Verification items for the finished model (mm, model axes). Coordinates: 2 decimals unless noted, no trailing zeros. Write each loop counter-clockwise with the first axis right and the second up, starting at its lowest first coordinate (ties: lowest second). Pieces come first, ordered by that corner, then holes. Notation, with made-up numbers: (67.5, 79) - (106.5, 79) arc R7 cw to (106.5, 92) - close; hole circle Ø1 at (44, -20.5). An arc over 180 degrees is marked (long way). Use CSV: the item, a comma, the result in double quotes. Start each with the question number.
```python
from build123d import *

# Parameters (mm, degrees)
F0_R     = 15
F0_R_2   = 22.5
F1_DEPTH = 15
F2_DEPTH = 15.001
F3_R     = 3
F4_DEPTH = 25


with BuildPart() as f1:
    # F0 (on Front) → F1 (new body)
    with BuildSketch(Plane.XZ):
        Circle(F0_R)
        Circle(F0_R_2)
        Circle(F0_R, mode=Mode.SUBTRACT)
    extrude(amount=-F1_DEPTH)

    # F0 (on Front) → F2 (cut, through all)
    with BuildSketch(Plane.XZ):
        Circle(F0_R)
    extrude(amount=-F2_DEPTH, mode=Mode.SUBTRACT)

    # F3 (on Top) → F4 (cut, symmetric)
    with BuildSketch(Plane.XY):
        with Locations((0, 7.5)):
            Circle(F3_R)
    extrude(amount=F4_DEPTH, both=True, mode=Mode.SUBTRACT)


solid = f1.part
```
Q1. Release check for a two-part mould opening along Z. For faces 1 (the cylindrical face through (10.382, 7.395, -19.961)), 2 (the cylindrical face through (-3.252, 7.395, -14.643)), 3 (the cylindrical face through (-3, 7.6, 18.7)) record: released by +Z, released by -Z, zero draft, split by the parting line, or undercut.
Q2. Cross-section at A-A (z = 0). Record the cut outline in (x, y), plus the area to 3 significant figures.
Q3. Cross-section at C-C (x = 0). Record the cut outline in (y, z), plus the area to 3 significant figures.
Q4. Cross-section at D-D (y = 2.75). Record the cut outline in (x, z).
Q5. Gauge pin test, flat ends, axial feed: pin 1 (1.5 mm diameter, centred on x = -16.5, y = 3, fed in from -Z); pin 2 (8 mm diameter, centred on x = -17.5, y = 8.5, fed in from +Z); pin 3 (4 mm diameter, centred on y = 8.5, z = -2.5, fed in from +X); pin 4 (8 mm diameter, centred on x = 10.5, z = -3, fed in from +Y). Record the tip position at first contact, or that the pin passes through.
Q6. Scan lines: line 1 along Y through (x, z) = (0, 17.75); line 2 along X through (y, z) = (7.5, -19); line 3 along Z through (x, y) = (-5, 12.75). Record each from-to range of solid material in increasing order. Write a range as from..to.
Q7. Cross-section at B-B (x = -5). Record the cut outline in (y, z).
Reply:
1,face 1,"split by the parting line"
1,face 2,"undercut"
1,face 3,"zero draft"
2,outline,"(-22.5, 0) - (-15, 0) - (-15, 15) - (-22.5, 15) - close; (15, 0) - (22.5, 0) - (22.5, 15) - (15, 15) - close"
2,area,"225 mm^2"
3,outline,"(0, -22.5) - (4.5, -22.5) - (4.5, -15) - (0, -15) - close; (0, 15) - (4.5, 15) - (4.5, 22.5) - (0, 22.5) - close; (10.5, -22.5) - (15, -22.5) - (15, -15) - (10.5, -15) - close; (10.5, 15) - (15, 15) - (15, 22.5) - (10.5, 22.5) - close"
3,area,"135 mm^2"
4,outline,"circle Ø45 at (0, 0); hole circle Ø30 at (0, 0)"
5,pin 1,"z = -16.07"
5,pin 2,"z = 18"
5,pin 3,"x = 22.49"
5,pin 4,"through"
6,line 1,"0..4.5, 10.5..15"
6,line 2,"-12.05..-3, 3..12.05"
6,line 3,"-21.94..-14.14, 14.14..21.94"
7,outline,"(0, -21.94) - (15, -21.94) - (15, -14.14) - (0, -14.14) - close; (0, 14.14) - (15, 14.14) - (15, 21.94) - (0, 21.94) - close"
